Input: dimensioned drawing with shaded views. Units: mm. Origin: part minimum x, y, z. A direction names the side the tool comes from. Coordinates: 2 decimals unless noted, no trailing zeros. Loops run counter-clockwise (first coordinate to the right, second up) from the corner with the lowest first, then second, coordinate; pieces in that order, holes last.
(1) Section D-D, the plane y = 40. Return loops of the section in (x, z), then the cut area to 3 significant figures.
(2) Contact query for flat-ended pins moving along their axis: P1, Ø10, axis at x = 37.5, y = 45.5, coming from the +Z side; P2, Ø2.5, axis at y = 46, z = 9, coming from the +X side; P3, Ø5.5, axis at x = 62.5, y = 26, coming from the +Z side. Output: stop coordinate, or through.
(3) Section B-B, the plane x = 38.1. Return loops of the section in (y, z).
(4) Section A-A, the plane z = 6.35. Return loops of the section in (x, y), then the cut area to 3 significant figures.
(5) Line query: L1, parallel to X at y = 15, z = 11.5; L2, parallel to X at y = 11.5, z = 11; L3, parallel to X at y = 25.4, z = 7.5. Output: solid intervals per line, ascending.
(6) Mould query, pull axis X, two halves, no side actions, for the marked faces 1, 2 and 3. Classes: released by +X, released by -X, zero draft, split by the parting line, or undercut.
(7) Set-up query: the marked faces 4, 5 and 6. Return all of +Z, -Z, +X, -X, +Y, -Y with unobstructed straight access to the full face (end or side cutting, diameter ignored); none if empty.
(8) Section C-C, the plane y = 25.4. Return loops of the section in (x, z), then the cut area to 4 significant figures.
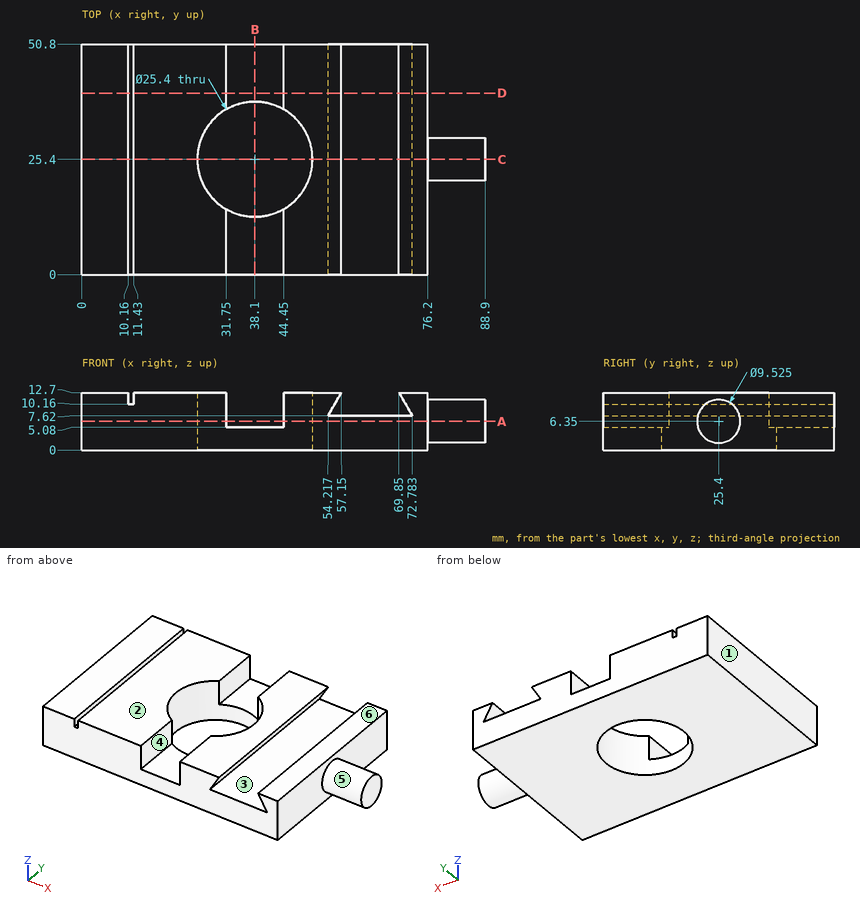
Report:
1. outline: (0, 0) - (76.2, 0) - (76.2, 12.7) - (69.85, 12.7) - (72.78, 7.62) - (54.22, 7.62) - (57.15, 12.7) - (44.45, 12.7) - (44.45, 5.08) - (31.75, 5.08) - (31.75, 12.7) - (11.43, 12.7) - (11.43, 10.16) - (10.16, 10.16) - (10.16, 12.7) - (0, 12.7) - close
1. area: 788 mm2
2. P1: stops at z = 5.08
2. P2: stops at x = 76.2
2. P3: stops at z = 7.62
3. outline: (0, 0) - (12.7, 0) - (12.7, 5.08) - (0, 5.08) - close; (38.1, 0) - (50.8, 0) - (50.8, 5.08) - (38.1, 5.08) - close
4. outline: (0, 0) - (31.75, 0) - (31.75, 14.4) arc R12.7 cw to (31.75, 36.4) - (31.75, 50.8) - (0, 50.8) - close; (44.45, 0) - (76.2, 0) - (76.2, 20.64) - (88.9, 20.64) - (88.9, 30.16) - (76.2, 30.16) - (76.2, 50.8) - (44.45, 50.8) - (44.45, 36.4) arc R12.7 cw to (44.45, 14.4) - close
4. area: 3,150 mm2
5. L1: x = 0 to 10.16, 11.43 to 30.81, 45.39 to 56.46, 70.54 to 76.2
5. L2: x = 0 to 10.16, 11.43 to 31.75, 44.45 to 56.17, 70.83 to 76.2
5. L3: x = 0 to 25.4, 50.8 to 88.9
6. face 1: released by -X
6. face 2: zero draft
6. face 3: undercut
7. face 4: +Z, +Y, -Y
7. face 5: +X
7. face 6: +Z, +X, -X, +Y, -Y
8. outline: (0, 0) - (25.4, 0) - (25.4, 12.7) - (11.43, 12.7) - (11.43, 10.16) - (10.16, 10.16) - (10.16, 12.7) - (0, 12.7) - close; (50.8, 0) - (76.2, 0) - (76.2, 1.59) - (88.9, 1.59) - (88.9, 11.11) - (76.2, 11.11) - (76.2, 12.7) - (69.85, 12.7) - (72.78, 7.62) - (54.22, 7.62) - (57.15, 12.7) - (50.8, 12.7) - close
8. area: 683.5 mm2
